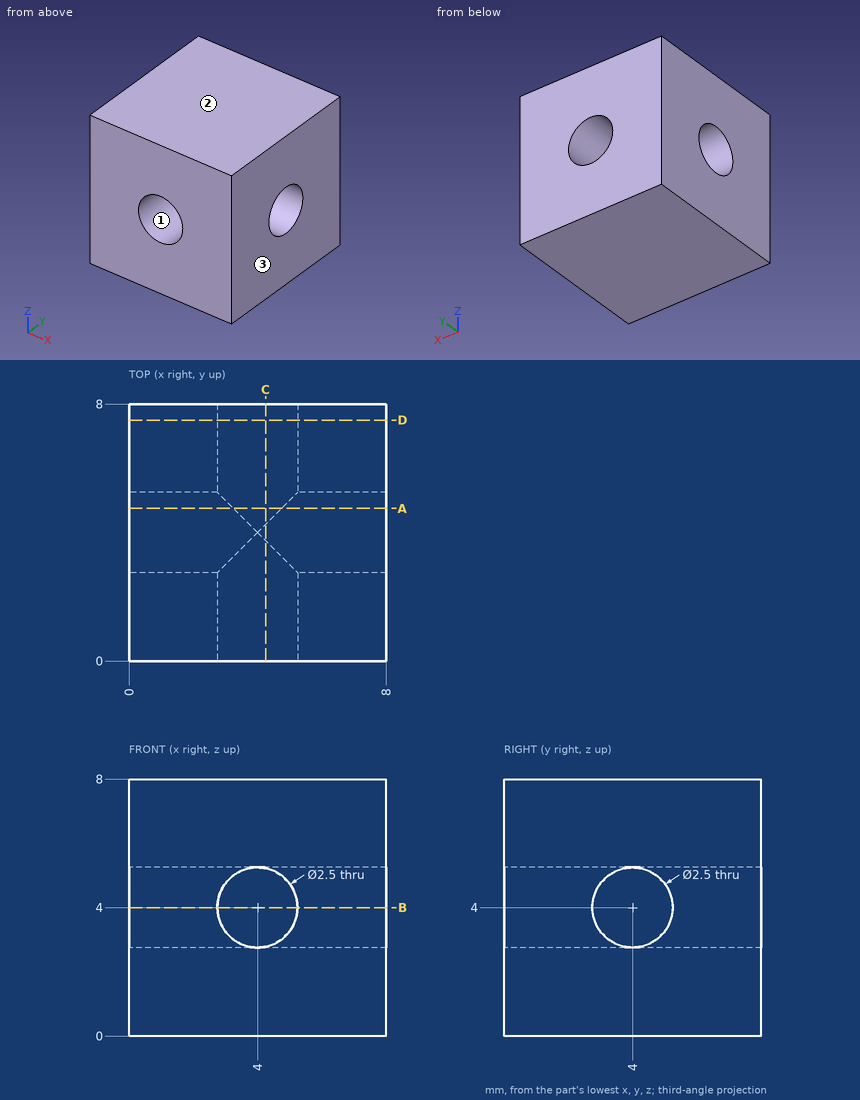
Drawing for the job (mm, zero at the part's lowest x, y, z). Coordinates: 2 decimals unless noted, no trailing zeros. Write each loop counter-clockwise with the first axis right and the second up, starting at its lowest first coordinate (ties: lowest second). Pieces come first, ordered by that corner, then holes. Notation, with made-up numbers: (38.5, -33) - (63.5, -33) arc R20 cw to (63.5, 1) - close; hole circle Ø4 at (51, 28). An arc over 180 degrees is marked (long way). Write each question's results on one line, items separated by ' | '. Start each with the question number.
1) Cut at A-A (y = 4.75). Write the cut outline in (x, z), then the cut area to 3 significant figures.
2) Mould opens along X. For the marked faces 1, 2 and 3 say: pulls with the +X half, pulls with the -X half, needs draft (parallel to the pull), parting line crosses it, or undercut.
3) Cut at D-D (y = 7.5). Write the cut outline in (x, z).
4) Cut at C-C (x = 4.25). Write the cut outline in (y, z), then the cut area to 3 significant figures.
5) Probe line 1 along Z through (x, y) = (4, 1.75). List the from-to ranges inside material, lowest first. Write a range as from..to.
6) Flat gauge pin, fed straight in: P1, Ø2, axis at x = 4, z = 4, coming from the +Y side. Where does the tip first touch, or does it go through?
7) Cut at B-B (z = 4). Write the cut outline in (x, y).
Returned:
1) outline: (0, 0) - (8, 0) - (8, 3) - (4.75, 3) arc R1.25 cw to (3.25, 3) - (0, 3) - close; (0, 5) - (3.25, 5) arc R1.25 cw to (4.75, 5) - (8, 5) - (8, 8) - (0, 8) - close | area: 47.5 mm^2
2) face 1: undercut | face 2: needs draft | face 3: pulls with the +X half
3) outline: (0, 0) - (8, 0) - (8, 8) - (0, 8) - close; hole circle Ø2.5 at (4, 4)
4) outline: (0, 0) - (8, 0) - (8, 2.78) - (4.25, 2.78) arc R1.25 cw to (3.75, 2.78) - (0, 2.78) - close; (0, 5.22) - (3.75, 5.22) arc R1.25 cw to (4.25, 5.22) - (8, 5.22) - (8, 8) - (0, 8) - close | area: 44.4 mm^2
5) line 1: 0..2.75, 5.25..8
6) P1: through
7) outline: (0, 0) - (2.75, 0) - (2.75, 2.75) - (0, 2.75) - close; (0, 5.25) - (2.75, 5.25) - (2.75, 8) - (0, 8) - close; (5.25, 0) - (8, 0) - (8, 2.75) - (5.25, 2.75) - close; (5.25, 5.25) - (8, 5.25) - (8, 8) - (5.25, 8) - close
